Here's how the part is built. I have some questions about the finished solid (model axes, mm). Coordinates: 2 decimals unless noted, no trailing zeros. Loops run counter-clockwise (first coordinate to the right, second up) from the corner with the lowest first, then second, coordinate; pieces in that order, holes last. Notation, with made-up numbers: (31.25, 51.5) -> (41.25, 51.5) arc R27 ccw to (41.25, 80.5) -> close; hole circle Ø2 at (42, 46). An arc over 180 degrees is marked (long way). Answer as a JSON object with one key per item and string values. Group by question number.
1) I want a section at B-B (y = 10.5). Write out the boundary of the cut face in (x, z).
2) I need wall thicknesses on probe 1 along Z at (x, y) = (-44.45, 13.75); probe 2 along X at (y, z) = (13.5, -0.25); probe 3 along X at (y, z) = (14.75, 0.5). Which ranges of each line are inside material? Lowest first, please. Write a range as [from, to].
3) I want a section at A-A (x = -44.45). Write out the boundary of the cut face in (y, z) (1 decimal), then the cut area to 3 significant figures.
```python
from build123d import *

# Parameters (mm, degrees)
BOSS_EXTRUDE2_DEPTH                               = 22.225
BOSS_EXTRUDE2_DEPTH_BACK                          = 10
SKETCH2_W                                         = 153.14353988
SKETCH2_H                                         = 6.35
CUT_EXTRUDE1_DEPTH                                = 4.7625
SKETCH3_W                                         = 152.758434582
SKETCH3_H                                         = 6.35
CUT_EXTRUDE2_DEPTH                                = 4.7625
FILLET3_R                                         = 12.7
FILLET4_R                                         = 12.7
FILLET5_R                                         = 12.7
FILLET6_R                                         = 12.7
CUT_EXTRUDE3_DEPTH                                = 94.675
CUT_EXTRUDE3_DEPTH_BACK                           = 84.675
SKETCH12_R                                        = 168.402
CSK_FOR_8_FLAT_HEAD_SOCKET_CAP_SCREW2_D           = 4.4958
CSK_FOR_8_FLAT_HEAD_SOCKET_CAP_SCREW2_CSINK_D     = 9.1186
CSK_FOR_8_FLAT_HEAD_SOCKET_CAP_SCREW2_CSINK_ANGLE = 82
SKETCH25_W                                        = 151.836061676
SKETCH25_H                                        = 46.299624525
CUT_EXTRUDE4_DEPTH                                = 10.16
SKETCH26_W                                        = 138.514547674
SKETCH26_H                                        = 27.845278494
CUT_EXTRUDE5_DEPTH                                = 23.368


with BuildPart() as part:
    # Sketch1 → Boss-Extrude2 (new, two sides: drawn at the far end of the back side and taken through both)
    with BuildSketch(Plane(origin=(0, 0, 0), x_dir=(1, 0, 0), z_dir=(0, 1, 0)).offset(-BOSS_EXTRUDE2_DEPTH_BACK)):
        with BuildLine():
            Line((37.204956004, 9.525), (-37.204956004, 9.525))
            ThreePointArc((-37.204956004, 9.525), (-39.498289417, 9.316221792), (-41.716221563, 8.696751473))
            Line((-41.716221563, 8.696751473), (-62.649818949, 0.741984467))
            ThreePointArc((-62.649818949, 0.741984467), (-63.161614851, 0), (-62.649818949, -0.741984467))
            Line((-62.649818949, -0.741984467), (-41.716221563, -8.696751473))
            ThreePointArc((-41.716221563, -8.696751473), (-39.498289417, -9.316221792), (-37.204956004, -9.525))
            Line((-37.204956004, -9.525), (37.204956004, -9.525))
            ThreePointArc((37.204956004, -9.525), (39.498289417, -9.316221792), (41.716221563, -8.696751473))
            Line((41.716221563, -8.696751473), (62.649818949, -0.741984467))
            ThreePointArc((62.649818949, -0.741984467), (63.161614851, 0), (62.649818949, 0.741984467))
            Line((62.649818949, 0.741984467), (41.716221563, 8.696751473))
            ThreePointArc((41.716221563, 8.696751473), (39.498289417, 9.316221792), (37.204956004, 9.525))
        make_face()
    extrude(amount=BOSS_EXTRUDE2_DEPTH + BOSS_EXTRUDE2_DEPTH_BACK)

    # Sketch2 → Cut-Extrude1 (cut)
    with BuildSketch(Plane.XY.offset(9.525)):
        with Locations((7.894658594, 12.7)):
            Rectangle(SKETCH2_W, SKETCH2_H)
    extrude(amount=-CUT_EXTRUDE1_DEPTH, mode=Mode.SUBTRACT)

    # Sketch3 → Cut-Extrude2 (cut)
    with BuildSketch(Plane(origin=(0, 0, -9.525), x_dir=(-1, 0, 0), z_dir=(0, 0, -1))):
        with Locations((8.600684972, 12.7)):
            Rectangle(SKETCH3_W, SKETCH3_H)
    extrude(amount=-CUT_EXTRUDE2_DEPTH, mode=Mode.SUBTRACT)

    # Fillet3
    fillet3_edges = [part.edges().sort_by_distance(p)[0] for p in [
        (52.069514915, 12.7, -4.7625),
    ]]
    fillet(fillet3_edges, radius=FILLET3_R)

    # Fillet4
    fillet4_edges = [part.edges().sort_by_distance(p)[0] for p in [
        (52.069514915, 12.7, 4.7625),
    ]]
    fillet(fillet4_edges, radius=FILLET4_R)

    # Fillet5
    fillet5_edges = [part.edges().sort_by_distance(p)[0] for p in [
        (-52.069514915, 12.7, 4.7625),
    ]]
    fillet(fillet5_edges, radius=FILLET5_R)

    # Fillet6
    fillet6_edges = [part.edges().sort_by_distance(p)[0] for p in [
        (-52.069514915, 12.7, -4.7625),
    ]]
    fillet(fillet6_edges, radius=FILLET6_R)

    # Sketch12 → Cut-Extrude3 (cut, two sides: drawn at the far end of the back side and taken through both)
    with BuildSketch(Plane(origin=(0, 0, 0), x_dir=(0, 0, -1), z_dir=(1, 0, 0)).offset(-CUT_EXTRUDE3_DEPTH_BACK)):
        with Locations((0, -168.402)):
            Circle(SKETCH12_R)
    extrude(amount=CUT_EXTRUDE3_DEPTH + CUT_EXTRUDE3_DEPTH_BACK, mode=Mode.SUBTRACT)

    # CSK for #8 Flat Head Socket Cap Screw2 (through all)
    with Locations(Plane(origin=(0, 22.225, 0), x_dir=(1, 0, 0), z_dir=(0, 1, 0))):
        with Locations((-44.45, 0), (44.45, 0)):
            CounterSinkHole(CSK_FOR_8_FLAT_HEAD_SOCKET_CAP_SCREW2_D / 2, CSK_FOR_8_FLAT_HEAD_SOCKET_CAP_SCREW2_CSINK_D / 2, counter_sink_angle=CSK_FOR_8_FLAT_HEAD_SOCKET_CAP_SCREW2_CSINK_ANGLE)

    # Sketch25 → Cut-Extrude4 (cut)
    with BuildSketch(Plane(origin=(0, 15.875, 0), x_dir=(1, 0, 0), z_dir=(0, 1, 0))):
        with Locations((2.779627567, -6.342868994)):
            Rectangle(SKETCH25_W, SKETCH25_H)
    extrude(amount=CUT_EXTRUDE4_DEPTH, mode=Mode.SUBTRACT)

    # Sketch26 → Cut-Extrude5 (cut)
    with BuildSketch(Plane(origin=(0, 9.525, 0), x_dir=(1, 0, 0), z_dir=(0, 1, 0))):
        with Locations((0.08280518, -0.921909218)):
            Rectangle(SKETCH26_W, SKETCH26_H)
    extrude(amount=-CUT_EXTRUDE5_DEPTH, mode=Mode.SUBTRACT)


solid = part.part
```
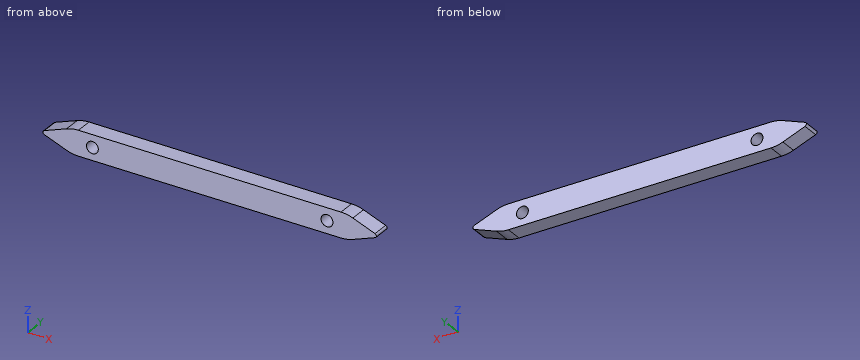
Determined:
{
 "1": {"outline": "(-62.65, -0.74) -> (-54.25, -3.93) arc R12.7 ccw to (-49.74, -4.76) -> (49.74, -4.76) arc R12.7 ccw to (54.25, -3.93) -> (62.65, -0.74) arc R0.79 ccw to (62.65, 0.74) -> (54.25, 3.93) arc R12.7 ccw to (49.74, 4.76) -> (-49.74, 4.76) arc R12.7 ccw to (-54.25, 3.93) -> (-62.65, 0.74) arc R0.79 ccw to start; hole circle Ø4.5 at (-44.45, 0); hole circle Ø4.5 at (44.45, 0)"},
 "2": {"probe 1": "[-4.76, -2.25], [2.25, 4.76]", "probe 2": "[-63.12, -46.68], [-42.22, 42.22], [46.68, 63.12]", "probe 3": "[-62.98, -46.64], [-42.26, 42.26], [46.64, 62.98]"},
 "3": {"outline": "(9.5, -4.8) -> (15.9, -4.8) -> (15.9, -2.2) -> (9.5, -2.2) -> close; (9.5, 2.2) -> (15.9, 2.2) -> (15.9, 4.8) -> (9.5, 4.8) -> close", "area": "31.9 mm^2"}
}
